Autodesk Inventor part; units mm, degrees
ref_plane "YZ Plane" through (0, 0, 0) normal (1, 0, 0) x (0, 1, 0)
ref_plane "XZ Plane" through (0, 0, 0) normal (0, 1, 0) x (-1, 0, 0)
ref_plane "XY Plane" through (0, 0, 0) normal (0, 0, 1) x (1, 0, 0)
sketch "Sketch1" plane through (0, 0, 0) normal (1, 0, 0) x (0, 1, 0)
  line L0 (0, -1.4986) -> (-1.2978, -0.7493)
  line L1 (-1.2978, -0.7493) -> (-1.2978, 0.7493)
  line L2 (-1.2978, 0.7493) -> (0, 1.4986)
  line L3 (0, 1.4986) -> (1.2978, 0.7493)
  line L4 (1.2978, 0.7493) -> (1.2978, -0.7493)
  line L5 (1.2978, -0.7493) -> (0, -1.4986)
  line L6 (1.9295, -1.114) -> (1.9295, 1.114)
  line L7 (1.9295, 1.114) -> (0, 2.228)
  line L8 (0, 2.228) -> (-1.9295, 1.114)
  line L9 (-1.9295, 1.114) -> (-1.9295, -1.114)
  line L10 (-1.9295, -1.114) -> (0, -2.228)
  line L11 (0, -2.228) -> (1.9295, -1.114)
  point P0 (0, 0)
  point P1 (0, 0)
  dimension "d0" = 1.4986
extrude "Extrusion1" add sketch "Sketch1" along normal blind 25.4
properties part number "Metal Fastener"
Design review of the part built by this model. Coordinates are the model's own, in mm. A direction names the side the tool comes from. Round coordinates to 2 decimals unless told otherwise and drop trailing zeros. Write each loop counter-clockwise with the first axis right and the second up, starting at its lowest first coordinate (ties: lowest second). Pieces come first, ordered by that corner, then holes.
Item 1: Consider section A-A on z = 0.3. Give the boundary of the cut face in (x, y), and give its area (3 significant figures).
Item 2: Draft analysis for pull direction Z (two halves, no side actions). For faces 3 (the flat face through (13, -1.298, 0)), 4 (the flat face through (12.52, -0.98, -1.66)), 5 (the flat face through (12.522, -0.658, 1.119)), 6 (the flat face through (13, -1.93, 0)), state which applies: released by +Z, released by -Z, zero draft, split by the parting line, or undercut.
Item 3: Consider section B-B on x = 5.25. Give the boundary of the cut face in (y, z).
Item 4: For faces 1 (the flat face through (12.522, 0.658, -1.119)), 2 (the flat face through (25.4, -0.5, -1.5)), list the 3-axis set-ups (+Z, -Z, +X, -X, +Y, -Y) from which the entire face can be reached by the end or side of a thin tool; tool diameter is ignored.
Item 5: Consider section C-C on y = 0.8. Give the boundary of the cut face in (x, z).
Item 6: Wall thickness on L1, parallel to Y at x = 10.5, z = -0.3; L2, parallel to Z at x = 16, y = -0.4; L3, parallel to Z at x = 24, y = 1.15: over which ranges is each line inside the solid? List them lowest first.
Check values:
1. outline: (0, -1.93) - (25.4, -1.93) - (25.4, -1.3) - (0, -1.3) - close; (0, 1.3) - (25.4, 1.3) - (25.4, 1.93) - (0, 1.93) - close
1. area: 32.1 mm2
2. face 3: undercut
2. face 4: released by -Z
2. face 5: undercut
2. face 6: zero draft
3. outline: (-1.93, -1.11) - (0, -2.23) - (1.93, -1.11) - (1.93, 1.11) - (0, 2.23) - (-1.93, 1.11) - close; hole (-1.3, -0.75) - (0, -1.5) - (1.3, -0.75) - (1.3, 0.75) - (0, 1.5) - (-1.3, 0.75) - close
4. face 1: +X, -X
4. face 2: +Z, -Z, +X, +Y, -Y
5. outline: (0, -1.77) - (25.4, -1.77) - (25.4, -1.04) - (0, -1.04) - close; (0, 1.04) - (25.4, 1.04) - (25.4, 1.77) - (0, 1.77) - close
6. L1: y = -1.93 to -1.3, 1.3 to 1.93
6. L2: z = -2 to -1.27, 1.27 to 2
6. L3: z = -1.56 to -0.83, 0.83 to 1.56
